Geometry: final body of the model. Coordinates: model frame, mm. Coordinates: 2 decimals unless noted, no trailing zeros. Write each loop counter-clockwise with the first axis right and the second up, starting at its lowest first coordinate (ties: lowest second). Pieces come first, ordered by that corner, then holes. Notation, with made-up numbers: (-5, 83) - (7, 83) arc R34 cw to (7, 114) - close; hole circle Ø7 at (45.5, 25.25). An arc over 180 degrees is marked (long way). Answer as a JSON object with one key per item and string values. Group by question number.
Item 1: Section A-A on y = 134. Return loops of the section in (x, z).
Item 2: Section D-D on x = -27. Return loops of the section in (y, z) (3 decimals).
Item 3: Section B-B on x = 15.5. Return loops of the section in (y, z), and give its area (3 significant figures).
Item 4: Section C-C on x = 61. Return loops of the section in (y, z), and give its area (3 significant figures).
Item 5: First-contact query: pin 1 Ø4 at (x, y) = (-35, 156.1) entering from +Z; pin 2 Ø0.6 at (x, z) = (47, 1) entering from -Y; pin 3 Ø1 at (x, z) = (43, 0.5) entering from +Y. Flat tips, straight axial feed; report the tip coordinate or a pass-through.
Item 6: Line query: line 1 along X through (y, z) = (156.1, 1.6); line 2 along X through (y, z) = (86, 1.4); line 3 along Y through (x, z) = (53, 0.65). Output: solid intervals per line, ascending. Write a range as from..to.
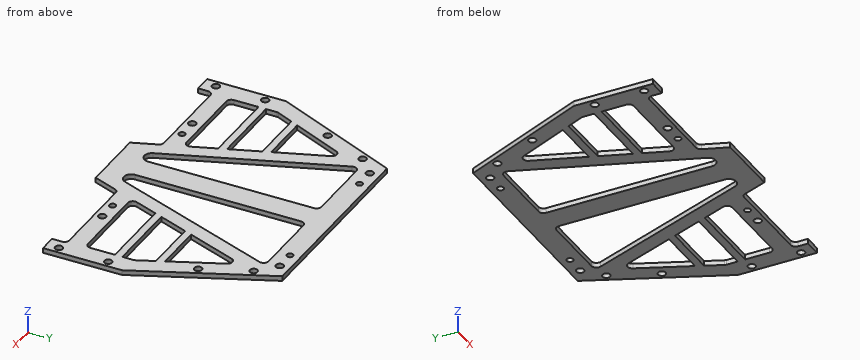
```python
from build123d import *

# Parameters (mm, degrees)
SKETCH_1_R          = 40.9
SKETCH_1_R_2        = 1.525
EXTRUDE_1_DEPTH     = 2
EXTRUDE_2_DEPTH     = 2
SKETCH_4_R          = 1.55
CUT_EXTRUDE_2_DEPTH = 10
SKETCH_5_OUTSIDE_W  = 183.288
SKETCH_5_OUTSIDE_H  = 259.388
CUT_EXTRUDE_3_DEPTH = 10
SKETCH_7_R          = 1.3
SKETCH_7_R_2        = 1.55
CUT_EXTRUDE_4_DEPTH = 10
CUT_EXTRUDE_5_DEPTH = 10
SKETCH_9_W          = 25.793449444
SKETCH_9_H          = 3
SKETCH_9_W_2        = 31.374844792
EXTRUDE_4_DEPTH     = 2
SKETCH_12_W         = 20
SKETCH_12_H         = 5
CUT_EXTRUDE_7_DEPTH = 10


with BuildPart() as part:
    # 草图1 → 凸台-拉伸1 (new body)
    with BuildSketch(Plane.XY):
        with BuildLine():
            Line((-48, 105.1), (48, 105.1))
            Line((48, 105.1), (66, 105.1))
            Line((66, 105.1), (66, 52.6))
            Line((66, 52.6), (45.955327857, -13.860297311))
            ThreePointArc((45.955327857, -13.860297311), (0, -48), (-45.955327857, -13.860297311))
            Line((-45.955327857, -13.860297311), (-66, 52.6))
            Line((-66, 52.6), (-66, 105.1))
            Line((-66, 105.1), (-48, 105.1))
        make_face()
        Circle(SKETCH_1_R, mode=Mode.SUBTRACT)
        with Locations((12.835117837, 41.981778787)):
            Circle(SKETCH_1_R_2, mode=Mode.SUBTRACT)
        with Locations((-17.153096541, 40.410163067)):
            Circle(SKETCH_1_R_2, mode=Mode.SUBTRACT)
        with Locations((-31.749094475, 31.749094475)):
            Circle(SKETCH_1_R_2, mode=Mode.SUBTRACT)
        with Locations((31.749094475, 31.749094475)):
            Circle(SKETCH_1_R_2, mode=Mode.SUBTRACT)
        with Locations((31.749094475, -31.749094475)):
            Circle(SKETCH_1_R_2, mode=Mode.SUBTRACT)
        with Locations((-31.749094475, -31.749094475)):
            Circle(SKETCH_1_R_2, mode=Mode.SUBTRACT)
        with Locations((-9.5, 52.6)):
            Circle(SKETCH_1_R_2, mode=Mode.SUBTRACT)
        with Locations((9.5, 52.6)):
            Circle(SKETCH_1_R_2, mode=Mode.SUBTRACT)
    extrude(amount=EXTRUDE_1_DEPTH)

    # 草图3 → 凸台-拉伸2 (add)
    with BuildSketch(Plane.XY.offset(2)):
        Polygon((-66, 105.1), (-42, 160.1), (-22, 160.1), (22, 160.1), (42, 160.1), (66, 105.1), (22, 105.1), (-22, 105.1), align=None)
    extrude(amount=-EXTRUDE_2_DEPTH)

    # 草图4 → 切除-拉伸2 (cut)
    with BuildSketch(Plane.XY.offset(2)):
        with Locations((-61, 100.1)):
            Circle(SKETCH_4_R)
        with Locations((-61, 80.1)):
            Circle(SKETCH_4_R)
        with Locations((-42.333287047, 149.334828392)):
            Circle(SKETCH_4_R)
        with Locations((-50.332176167, 131.004040825)):
            Circle(SKETCH_4_R)
        with Locations((61, 80.1)):
            Circle(SKETCH_4_R)
        with Locations((61, 100.1)):
            Circle(SKETCH_4_R)
        with Locations((50.332176167, 131.004040825)):
            Circle(SKETCH_4_R)
        with Locations((42.333287047, 149.334828392)):
            Circle(SKETCH_4_R)
    extrude(amount=-CUT_EXTRUDE_2_DEPTH, mode=Mode.SUBTRACT)

    # 草图5 outside → 切除-拉伸3 (cut)
    with BuildSketch(Plane.XY.offset(2)):
        with Locations((0, 56.05)):
            Rectangle(SKETCH_5_OUTSIDE_W, SKETCH_5_OUTSIDE_H)
        Polygon((-40.690727285, 160.1), (-63.8, 107.141250029), (-63.8, 70.1), (63.8, 70.1), (63.8, 107.141250029), (40.690727285, 160.1), align=None, mode=Mode.SUBTRACT)
    extrude(amount=-CUT_EXTRUDE_3_DEPTH, mode=Mode.SUBTRACT)

    # 草图7 → 切除-拉伸4 (cut)
    with BuildSketch(Plane(origin=(0, 0, 0), x_dir=(-1, 0, 0), z_dir=(0, 0, -1))):
        with Locations((-27, 156.1)):
            Circle(SKETCH_7_R)
        with Locations((27, 156.1)):
            Circle(SKETCH_7_R)
        with Locations((-27, 84.1)):
            Circle(SKETCH_7_R)
        with Locations((27, 84.1)):
            Circle(SKETCH_7_R)
        with Locations((-35, 156.1)):
            Circle(SKETCH_7_R_2)
        with Locations((35, 156.1)):
            Circle(SKETCH_7_R_2)
        with Locations((-35, 84.1)):
            Circle(SKETCH_7_R_2)
        with Locations((35, 84.1)):
            Circle(SKETCH_7_R_2)
    extrude(amount=-CUT_EXTRUDE_4_DEPTH, mode=Mode.SUBTRACT)

    # 草图8 → 切除-拉伸5 (cut)
    with BuildSketch(Plane(origin=(0, 0, 0), x_dir=(-1, 0, 0), z_dir=(0, 0, -1))):
        with BuildLine():
            Line((-34.121847489, 151.1), (-7, 151.1))
            ThreePointArc((-7, 151.1), (-5.585786438, 150.514213562), (-5, 149.1))
            Line((-5, 149.1), (-5, 81.76505231))
            ThreePointArc((-5, 81.76505231), (-7.468491138, 78.812511315), (-10.811665553, 80.718851174))
            Line((-10.811665553, 80.718851174), (-35.996291191, 148.402532576))
            ThreePointArc((-35.996291191, 148.402532576), (-35.764244342, 150.241285493), (-34.121847489, 151.1))
        make_face()
        with BuildLine():
            Line((-38.719517417, 138.516098438), (-20.963747737, 90.797467424))
            ThreePointArc((-20.963747737, 90.797467424), (-21.195794586, 88.958714507), (-22.83819144, 88.1))
            Line((-22.83819144, 88.1), (-53.8, 88.1))
            ThreePointArc((-53.8, 88.1), (-55.214213562, 88.685786438), (-55.8, 90.1))
            Line((-55.8, 90.1), (-55.8, 107.554791913))
            ThreePointArc((-55.8, 107.554791913), (-55.757825007, 107.963351875), (-55.633078757, 108.354680825))
            Line((-55.633078757, 108.354680825), (-42.427039876, 138.618519926))
            ThreePointArc((-42.427039876, 138.618519926), (-40.538731553, 139.817868293), (-38.719517417, 138.516098438))
        make_face()
        with BuildLine():
            Line((-56.8, 79.1), (-56.8, 67.1))
            ThreePointArc((-56.8, 67.1), (-56.214213562, 65.685786438), (-54.8, 65.1))
            Line((-54.8, 65.1), (-14.280051905, 65.1))
            ThreePointArc((-14.280051905, 65.1), (-12.637655051, 65.958714507), (-12.405608203, 67.797467424))
            Line((-12.405608203, 67.797467424), (-16.870724482, 79.797467424))
            ThreePointArc((-16.870724482, 79.797467424), (-17.603882691, 80.742396853), (-18.745168184, 81.1))
            Line((-18.745168184, 81.1), (-54.8, 81.1))
            ThreePointArc((-54.8, 81.1), (-56.214213562, 80.514213562), (-56.8, 79.1))
        make_face()
        with BuildLine():
            Line((18.745168184, 81.1), (54.8, 81.1))
            ThreePointArc((54.8, 81.1), (56.214213562, 80.514213562), (56.8, 79.1))
            Line((56.8, 79.1), (56.8, 67.1))
            ThreePointArc((56.8, 67.1), (56.214213562, 65.685786438), (54.8, 65.1))
            Line((54.8, 65.1), (14.280051905, 65.1))
            ThreePointArc((14.280051905, 65.1), (12.637655051, 65.958714507), (12.405608203, 67.797467424))
            Line((12.405608203, 67.797467424), (16.870724482, 79.797467424))
            ThreePointArc((16.870724482, 79.797467424), (17.603882691, 80.742396853), (18.745168184, 81.1))
        make_face()
        with BuildLine():
            Line((55.633078757, 108.354680825), (42.427039876, 138.618519926))
            ThreePointArc((42.427039876, 138.618519926), (40.538731553, 139.817868293), (38.719517417, 138.516098438))
            Line((38.719517417, 138.516098438), (20.963747737, 90.797467424))
            ThreePointArc((20.963747737, 90.797467424), (21.195794586, 88.958714507), (22.83819144, 88.1))
            Line((22.83819144, 88.1), (53.8, 88.1))
            ThreePointArc((53.8, 88.1), (55.214213562, 88.685786438), (55.8, 90.1))
            Line((55.8, 90.1), (55.8, 107.554791913))
            ThreePointArc((55.8, 107.554791913), (55.757825007, 107.963351875), (55.633078757, 108.354680825))
        make_face()
        with BuildLine():
            Line((10.811665553, 80.718851174), (35.996291191, 148.402532576))
            ThreePointArc((35.996291191, 148.402532576), (35.764244342, 150.241285493), (34.121847489, 151.1))
            Line((34.121847489, 151.1), (7, 151.1))
            ThreePointArc((7, 151.1), (5.585786438, 150.514213562), (5, 149.1))
            Line((5, 149.1), (5, 81.76505231))
            ThreePointArc((5, 81.76505231), (7.468491138, 78.812511315), (10.811665553, 80.718851174))
        make_face()
    extrude(amount=-CUT_EXTRUDE_5_DEPTH, mode=Mode.SUBTRACT)

    # 草图9 → 凸台-拉伸4 (add)
    with BuildSketch(Plane(origin=(0, 0, 0), x_dir=(-1, 0, 0), z_dir=(0, 0, -1))):
        with Locations((-42.903275278, 116.6)):
            Rectangle(SKETCH_9_W, SKETCH_9_H)
        with Locations((-40.112577604, 101.6)):
            Rectangle(SKETCH_9_W_2, SKETCH_9_H)
        with Locations((40.112577604, 101.6)):
            Rectangle(SKETCH_9_W_2, SKETCH_9_H)
        with Locations((42.903275278, 116.6)):
            Rectangle(SKETCH_9_W, SKETCH_9_H)
    extrude(amount=-EXTRUDE_4_DEPTH)

    # 草图12 → 切除-拉伸7 (cut)
    with BuildSketch(Plane(origin=(0, 0, 0), x_dir=(-1, 0, 0), z_dir=(0, 0, -1))):
        with Locations((-53.8, 72.6)):
            Rectangle(SKETCH_12_W, SKETCH_12_H)
        with Locations((53.8, 72.6)):
            Rectangle(SKETCH_12_W, SKETCH_12_H)
    extrude(amount=-CUT_EXTRUDE_7_DEPTH, mode=Mode.SUBTRACT)


solid = part.part
```
Checks:
{
 "1": {"outline": "(-52.08, 0) - (-44.44, 0) - (-44.44, 2) - (-52.08, 2) - close; (-37.04, 0) - (-30.64, 0) - (-30.64, 2) - (-37.04, 2) - close; (-5, 0) - (5, 0) - (5, 2) - (-5, 2) - close; (30.64, 0) - (37.04, 0) - (37.04, 2) - (30.64, 2) - close; (44.44, 0) - (52.08, 0) - (52.08, 2) - (44.44, 2) - close"},
 "2": {"outline": "(81.1, 0) - (82.8, 0) - (82.8, 2) - (81.1, 2) - close; (85.4, 0) - (88.1, 0) - (88.1, 2) - (85.4, 2) - close; (100.1, 0) - (103.1, 0) - (103.1, 2) - (100.1, 2) - close; (107.02, 0) - (124.225, 0) - (124.225, 2) - (107.02, 2) - close; (151.1, 0) - (154.8, 0) - (154.8, 2) - (151.1, 2) - close; (157.4, 0) - (160.1, 0) - (160.1, 2) - (157.4, 2) - close"},
 "3": {"outline": "(76.11, 0) - (93.32, 0) - (93.32, 2) - (76.11, 2) - close; (151.1, 0) - (160.1, 0) - (160.1, 2) - (151.1, 2) - close", "area": "52.4 mm^2"},
 "4": {"outline": "(75.1, 0) - (78.55, 0) - (78.55, 2) - (75.1, 2) - close; (81.65, 0) - (98.55, 0) - (98.55, 2) - (81.65, 2) - close; (101.65, 0) - (113.56, 0) - (113.56, 2) - (101.65, 2) - close", "area": "64.5 mm^2"},
 "5": {"pin 1": "z = 2", "pin 2": "y = 81.1", "pin 3": "y = 155.95"},
 "6": {"line 1": "-42.44..-36.55, -33.45..-28.3, -25.7..25.7, 28.3..33.45, 36.55..42.44", "line 2": "-63.8..-12.78, -5..5, 12.78..63.8", "line 3": "81.1..88.1, 100.1..103.1, 114.39..131.89"}
}
